Source: CAD feature listing. Evaluate the final solid. Frame: model axes, mm. A direction names the side the tool comes from. Round coordinates to 2 decimals unless told otherwise and drop trailing zeros. Loops run counter-clockwise (first coordinate to the right, second up) from the corner with the lowest first, then second, coordinate; pieces in that order, holes last. Notation, with made-up numbers: (64.5, 79.25) -> (110.5, 79.25) arc R13 ccw to (110.5, 104.25) -> close; hole circle Ø2 at (6, -31.75). An arc over 180 degrees is marked (long way). Write item = value, one per line.
Autodesk Inventor part; units mm, degrees
ref_plane "YZ Plane" through (0, 0, 0) normal (1, 0, 0) x (0, 1, 0)
ref_plane "XZ Plane" through (0, 0, 0) normal (0, 1, 0) x (-1, 0, 0)
ref_plane "XY Plane" through (0, 0, 0) normal (0, 0, 1) x (1, 0, 0)
sketch "スケッチ1" plane through (0, 0, 0) normal (0, 0, 1) x (1, 0, 0)
  line L0 (0, 0) -> (15, 0)
  line L1 (15, 0) -> (15, 15)
  line L2 (15, 15) -> (0, 15)
  line L3 (0, 15) -> (0, 0)
  dimension "d0" = 15
  dimension "d1" = 15
extrude "押し出し1" add sketch "スケッチ1" along normal blind 120
sketch "スケッチ2" plane through (0, 15, 0) normal (0, 1, 0) x (1, 0, 0)
  point P0 (0, 0)
sketch "スケッチ3" plane through (15, 0, 0) normal (1, 0, 0) x (0, 0, -1)
  line L0 (-120, 0) -> (-120, 15)
  line L1 (0, 0) -> (-120, 0)
  line L2 (0, 0) -> (0, 15)
  point P0 (-110, 7.5)
  point P1 (-100, 7.5)
  point P2 (-90, 7.5)
  point P3 (-30, 7.5)
  point P4 (-20, 7.5)
  point P5 (-10, 7.5)
  dimension "d4" = 10
  dimension "d5" = 7.5
  dimension "d6" = 10
  dimension "d7" = 10
  dimension "d8" = 7.5
  dimension "d9" = 7.5
  dimension "d10" = 7.5
  dimension "d11" = 30
  dimension "d12" = 20
  dimension "d13" = 7.5
  dimension "d14" = 7.5
  dimension "d15" = 10
hole "穴1" at (15, 7.5, 110) at (15, 7.5, 100) at (15, 7.5, 90) at (15, 7.5, 30) at (15, 7.5, 20) at (15, 7.5, 10) direction (-1, 0, 0) diameter 3.2 end through all
sketch "スケッチ4" plane through (0, 0, 120) normal (0, 0, 1) x (1, 0, 0)
  line L0 (1.5, 13.5) -> (13.5, 13.5)
  line L1 (13.5, 13.5) -> (13.5, 1.5)
  line L2 (13.5, 1.5) -> (1.5, 1.5)
  line L3 (1.5, 1.5) -> (1.5, 13.5)
  line L4 (15, 15) -> (0, 15)
  line L5 (0, 15) -> (0, 0)
  dimension "d23" = 12
  dimension "d24" = 12
  dimension "d25" = 1.5
  dimension "d26" = 1.5
extrude "押し出し2" cut sketch "スケッチ4" against normal blind 600
properties part number "射出_角柱12" material "アルミニウム 6061"
1. Set-up query: faces 4 (the face through (7, 13.5, 61)), 5 (the face through (14, 8, 0)). Return all of +Z, -Z, +X, -X, +Y, -Y with unobstructed straight access to the full face (end or side cutting, diameter ignored); none if empty.
Evaluation:
face_4 = +Z, -Z
face_5 = -Z, +X, -X, +Y, -Y
2. Contact query for a flat-ended pin moving along its axis: pin 1 Ø1.5 at (x, z) = (6, 18) entering from -Y. Output: stop coordinate, or through.
Evaluation:
pin_1 = 0
3. Section query A-A (x = 6.75). Return the cut outline in (y, z).
Evaluation:
outline = (0, 0) -> (1.5, 0) -> (1.5, 120) -> (0, 120) -> close; (13.5, 0) -> (15, 0) -> (15, 120) -> (13.5, 120) -> close
4. Section query D-D (z = 54). Return the cut outline in (x, y).
Evaluation:
outline = (0, 0) -> (15, 0) -> (15, 15) -> (0, 15) -> close; hole (1.5, 1.5) -> (13.5, 1.5) -> (13.5, 13.5) -> (1.5, 13.5) -> close
5. Mould query, pull axis X, two halves, no side actions, for faces 1 (the face through (0, 8, 59)), 2 (the face through (14.24, 8.47, 11.27)), 3 (the face through (1.5, 7, 61)). Classes: released by +X, released by -X, zero draft, split by the parting line, or undercut.
Evaluation:
face_1 = released by -X
face_2 = zero draft
face_3 = undercut
6. Section query C-C (z = 110). Return the cut outline in (x, y).
Evaluation:
outline = (0, 0) -> (15, 0) -> (15, 5.9) -> (13.5, 5.9) -> (13.5, 1.5) -> (1.5, 1.5) -> (1.5, 5.9) -> (0, 5.9) -> close; (0, 9.1) -> (1.5, 9.1) -> (1.5, 13.5) -> (13.5, 13.5) -> (13.5, 9.1) -> (15, 9.1) -> (15, 15) -> (0, 15) -> close
7. Line query: probe 1 along X at (y, z) = (12, 95); probe 2 along Y at (x, z) = (13.9, 20). Output: solid intervals per line, ascending. Write a range as from..to.
Evaluation:
probe_1 = 0..1.5, 13.5..15
probe_2 = 0..5.9, 9.1..15
